Autodesk Inventor part; units mm, degrees
ref_plane "WorkPlane1" through (0, 0, 0) normal (0, 0, 1) x (1, 0, 0)
ref_plane "WorkPlane3" through (0, 0, -4.78) normal (0, 0, 1) x (1, 0, 0)
ref_plane "Work Plane3" through (0, -16.63, 0) normal (0, 1, 0) x (-1, 0, 0)
ref_plane "WorkPlane1" through (0, 0, 0) normal (0, 0, 1) x (1, 0, 0)
ref_plane "WorkPlane3" through (0, 0, -4.78) normal (0, 0, 1) x (1, 0, 0)
ref_plane "Work Plane3" through (0, -16.63, 0) normal (0, 1, 0) x (-1, 0, 0)
ref_plane "WorkPlane10" through (0, 16.63, 0) normal (0, 1, 0) x (-1, 0, 0)
sketch "Sketch1" plane through (0, 0, 0) normal (0, 0, 1) x (1, 0, 0)
  point P0 (0, 0)
sketch "Sketch2" plane through (0, 0, 0) normal (0, 0, 1) x (1, 0, 0)
  circle A0 centre (0, 0) radius 16.63
  dimension "d3" = 33.26
extrude "Extrusion1" add sketch "Sketch2" against normal blind 4.78
sketch "Sketch3" plane through (0, 0, -4.78) normal (0, 0, 1) x (1, 0, 0)
  point P0 (0, 0)
sketch "Sketch4" plane through (0, 0, 0) normal (0, 0, 1) x (1, 0, 0)
  circle A0 centre (0, 0) radius 16.63
hole "Hole1" at (0, 0, 0) direction (0, 0, -1) diameter 20.66 end through all
sketch "Sketch5" plane through (0, 16.63, 0) normal (0, 1, 0) x (-1, 0, 0)
  line L0 (-0.2453, 0) -> (-1.4403, 0)
  line L1 (0.5975, -4.78) -> (-0.2453, 0)
  line L2 (-0.5975, -4.78) -> (0.5975, -4.78)
  line L3 (-1.4403, 0) -> (-0.5975, -4.78)
  line L4 (-10.33, 0) -> (10.33, 0) construction
  line L5 (16.63, -4.78) -> (-16.63, -4.78) construction
  line L6 (0, -5.736) -> (0, 0.956)
  dimension "d15" = 80
  dimension "d18" = 0.5975
  dimension "d19" = 0.5975
extrude "Extrusion2" cut sketch "Sketch5" against normal blind 16.63
ref_plane "MSC_PT1" through (0, 0, 0) normal (0, 0, 1) x (1, 0, 0)
ref_plane "MSC_PT2" through (0, 0, -4.78) normal (0, 0, -1) x (-1, 0, 0)
equation "\"d7\" = Diam1"
equation "\"d4\" = ParH"
equation "\"d18\" = 0.125 * ParH"
equation "\"d19\" = 0.125 * ParH"
equation "\"d16\" = 0.5 * Diam2"
equation "\"d3\" = Diam2"
equation "\"Diam2\" = 33.26"
equation "\"ParH\" = 4.78"
equation "\"Diam1\" = 20.66"
equation "\"d20\" = 0.5 * Diam2"
properties part number "ASME B18.21.2M - 20" material "Steel, Mild"
Geometry check sheet. Reference: the model listing, model coordinates, mm. A direction names the side the tool comes from. Coordinates: 2 decimals unless noted, no trailing zeros. Loops run counter-clockwise (first coordinate to the right, second up) from the corner with the lowest first, then second, coordinate; pieces in that order, holes last. Notation, with made-up numbers: (65.25, -5) -> (88.25, -5) arc R25 cw to (88.25, 27) -> close; hole circle Ø9 at (-7.5, 31.5). An arc over 180 degrees is marked (long way). Put each result on its own line as item: value.
1) Cross-section at B-B on y = -5.5. Record the boundary of the cut face in (x, z), plus the area to 3 significant figures.
Result set:
outline: (-15.69, -4.78) -> (-8.74, -4.78) -> (-8.74, 0) -> (-15.69, 0) -> close; (8.74, -4.78) -> (15.69, -4.78) -> (15.69, 0) -> (8.74, 0) -> close
area: 66.4 mm^2
2) Release check for a two-part mould opening along X. For faces 3 (the flat face through (-8, -7, 0)), 4 (the flat face through (1.025, 13.469, -2.357)) record: released by +X, released by -X, zero draft, split by the parting line, or undercut.
Result set:
face 3: zero draft
face 4: undercut
3) Gauge pin test, flat end, axial feed: pin 1 Ø1.5 at (y, z) = (4, -1.5) entering from +X. Record the tip position at first contact, or that the pin passes through.
Result set:
pin 1: stops at x = 16.31
4) Tool access check on faces 1 (the flat face through (0, -11, -4.78)), 2 (the flat face through (-0.18, 13.52, -2.42)). Record the directions out of +Z, -Z, +X, -X, +Y, -Y that give a thin tool (end or side, any length) a straight path to the whole face; none if there is none.
Result set:
face 1: -Z, +X, -X, +Y, -Y
face 2: -Z, +Y
5) Cross-section at C-C on x = 11.5. Record the boundary of the cut face in (y, z), plus the area to 3 significant figures.
Result set:
outline: (-12.01, -4.78) -> (12.01, -4.78) -> (12.01, 0) -> (-12.01, 0) -> close
area: 115 mm^2
6) Cross-section at A-A on y = 1.5. Record the boundary of the cut face in (x, z).
Result set:
outline: (-16.56, -4.78) -> (-10.22, -4.78) -> (-10.22, 0) -> (-16.56, 0) -> close; (10.22, -4.78) -> (16.56, -4.78) -> (16.56, 0) -> (10.22, 0) -> close
7) Thickness scan on line 1 (X direction, y = 13, z = -1.5); line 2 (X direction, y = 1.5, z = -1.35); line 3 (Y direction, x = 6, z = -2.25). Record the ranges inside material, lowest first.
Result set:
line 1: x = -10.37 to -0.02, 1.18 to 10.37
line 2: x = -16.56 to -10.22, 10.22 to 16.56
line 3: y = -15.51 to -8.41, 8.41 to 15.51
8) Cross-section at D-D on z = -4.1. Record the boundary of the cut face in (x, y), plus the area to 3 significant figures.
Result set:
outline: (-0.48, 10.32) -> (-0.48, 16.62) arc R16.63 ccw (long way) to (0.72, 16.61) -> (0.72, 10.31) arc R10.33 cw (long way) to start
area: 526 mm^2
